```python
from build123d import *

# Parameters (mm, degrees)
SKETCH1_R           = 6.35
BOSS_EXTRUDE1_DEPTH = 12.7


with BuildPart() as part:
    # Sketch1 → Boss-Extrude1 (new body)
    with BuildSketch(Plane(origin=(0, 0, 0), x_dir=(1, 0, 0), z_dir=(0, 1, 0))):
        with BuildLine():
            Line((-0.068893261, 12.699813137), (304.731106739, 14.353275727))
            ThreePointArc((304.731106739, 14.353275727), (317.499813137, 1.722355851), (304.868893261, -11.046350547))
            Line((304.868893261, -11.046350547), (0.068893261, -12.699813137))
            ThreePointArc((0.068893261, -12.699813137), (-12.699813137, -0.068893261), (-0.068893261, 12.699813137))
        make_face()
        Circle(SKETCH1_R, mode=Mode.SUBTRACT)
        with Locations((304.8, 1.65346259)):
            Circle(SKETCH1_R, mode=Mode.SUBTRACT)
    extrude(amount=BOSS_EXTRUDE1_DEPTH)


solid = part.part
```
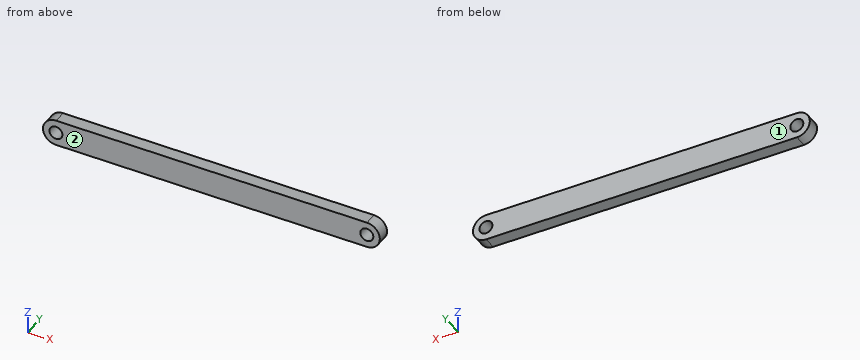
Here's how the part is built. I have some questions about the finished solid (model axes, mm). Face numbers are marked on the shaded views. Coordinates: 2 decimals unless noted, no trailing zeros. Loops run counter-clockwise (first coordinate to the right, second up) from the corner with the lowest first, then second, coordinate; pieces in that order, holes last. Notation, with made-up numbers: M 40.25,77 L 89.25,77 A20 cw 89.25,87 Z; hole C 27,39 d3. An arc over 180 degrees is marked long. One line per item, written item: value.
1. Will these pins go through, and if not, where does the flat tip stop? pin 1 Ø1.5 at (x, y) = (147, 2.5) entering from +Z; pin 2 Ø6 at (y, z) = (5.5, -7) entering from +X; pin 3 Ø4 at (x, y) = (121.5, 7) entering from +Z.
Geometry says:
pin 1: stops at z = 11.91
pin 2: stops at x = 317.28
pin 3: stops at z = 12.05
2. Imagine slicing it at A-A (y = 4.25). List the corners of the cut face in (x, z) for me.
Geometry says:
outline: M -0.07,-12.7 L 304.73,-14.35 A12.7 ccw 304.87,11.05 L 0.07,12.7 A12.7 ccw Z; hole C 0,0 d12.7; hole C 304.8,-1.65 d12.7
3. Imagine slicing it at B-B (x = 260.5). List the corners of the cut face in (y, z) for me.
Geometry says:
outline: M 0,-14.11 L 12.7,-14.11 L 12.7,11.29 L 0,11.29 Z
4. Thinking about a two-plate mould opening in Y: for the marked faces 1 and 2, which applies, +Y half, -Y half, draft (parallel to the pull), parting line (faces both ways), or undercut?
Geometry says:
face 1: +Y half
face 2: -Y half
5. Please list where these lines run through material, in increasing order: probe 1 along X at (y, z) = (5.75, -0.5); probe 2 along Z at (x, y) = (304.8, 5.5); probe 3 along X at (y, z) = (1.5, -3.5).
Geometry says:
probe 1: x = -12.69 to -6.33, 6.33 to 298.56, 311.04 to 317.45
probe 2: z = -14.35 to -8, 4.7 to 11.05
probe 3: x = -12.21 to -5.3, 5.3 to 298.72, 310.88 to 317.37
